from build123d import *

# Parameters (mm, degrees)
BOSS_EXTRUDE1_DEPTH = 20
SKETCH2_R           = 1.9
CUT_EXTRUDE1_DEPTH  = 7.5
CUT_EXTRUDE2_START  = -7.5
SKETCH3_R           = 1.9
CUT_EXTRUDE2_DEPTH  = 7.5


with BuildPart() as part:
    # Sketch1 → Boss-Extrude1 (new body)
    with BuildSketch(Plane(origin=(0, 0, 0), x_dir=(1, 0, 0), z_dir=(0, 1, 0))):
        Polygon((1.231025405, -2.055580158), (2.395697339, 0.038309195), (1.164671934, 2.093889353), (-1.231025405, 2.055580158), (-2.395697339, -0.038309195), (-1.164671934, -2.093889353), align=None)
    extrude(amount=BOSS_EXTRUDE1_DEPTH)

    # Sketch2 → Cut-Extrude1 (cut)
    with BuildSketch(Plane(origin=(0, 20, 0), x_dir=(1, 0, 0), z_dir=(0, 1, 0))):
        with Locations(Location((0, 0, 0), (0, 0, 270))):
            Circle(SKETCH2_R)
    extrude(amount=-CUT_EXTRUDE1_DEPTH, mode=Mode.SUBTRACT)

    # Sketch3 → Cut-Extrude2 (cut)
    with BuildSketch(Plane.XZ.offset(CUT_EXTRUDE2_START)):
        with Locations(Location((0, 0, 0), (0, 0, 90))):
            Circle(SKETCH3_R)
    extrude(amount=CUT_EXTRUDE2_DEPTH, mode=Mode.SUBTRACT)


solid = part.part
Source: CAD feature listing. Evaluate the final solid. Frame: model axes, mm. A direction names the side the tool comes from. Round coordinates to 2 decimals unless told otherwise and drop trailing zeros. Order: outer loops, then holes, each group sorted by start corner. A loop starts at its lowest first (then second) coordinate and runs counter-clockwise, first axis right, second up. Notation, with made-up numbers: (88.5, -32.75) - (109.5, -32.75) arc R23 cw to (109.5, -21.75) - close; hole circle Ø10 at (-20.5, 16.25). An arc over 180 degrees is marked (long way). Use a Markdown table: item, result. Add a question column.
1. Set-up query: faces 5 (the cylindrical face through (0.728, 3.802, 1.755)), 6 (the flat face through (-1.805, 9.86, -1.023)), 7 (the flat face through (0, 12.5, 0)). Return all of +Z, -Z, +X, -X, +Y, -Y with unobstructed straight access to the full face (end or side cutting, diameter ignored); none if empty.
2. Section query B-B (z = -1). Return the cut outline in (x, y).
3. Section query A-A (y = 17.75). Return the cut outline in (x, z).
4. Line query: probe 1 along Y at (x, z) = (-1, 0.1); probe 2 along X at (y, z) = (17, 0); probe 3 along X at (y, z) = (15.5, 0.35). Output: solid intervals per line, ascending.
5. Section query D-D (y = 10). Return the cut outline in (x, z).
6. Mould query, pull axis Z, two halves, no side actions, for faces 1 (the flat face through (0, 7.5, 0)), 2 (the flat face through (1.79, 9.86, -1.05)), 3 (the cylindrical face through (-0.728, 16.303, 1.755)), 4 (the flat face through (-1.79, 9.86, 1.05)). Classes: +Z half, -Z half, draft (parallel to the pull), parting line (faces both ways), or undercut.
7. Section query C-C (x = -0.75). Return the cut outline in (y, z).
8. First-contact query: pin 1 (1 mm diameter, centred on x = -0.5, y = 9.5, fed in from -Z); pin 2 (1.5 mm diameter, centred on y = 14.5, z = 1.5, fed in from -X). Flat tips, straight axial feed; report the tip coordinate or a pass-through.
Derived:
| question | item | result |
|---|---|---|
| 1 | face 5 | -Y |
| 1 | face 6 | -Z, -X, +Y, -Y |
| 1 | face 7 | +Y |
| 2 | outline | (-1.82, 0) - (-1.62, 0) - (-1.62, 7.5) - (1.62, 7.5) - (1.62, 0) - (1.82, 0) - (1.82, 20) - (1.62, 20) - (1.62, 12.5) - (-1.62, 12.5) - (-1.62, 20) - (-1.82, 20) - close |
| 3 | outline | (-2.4, 0.04) - (-1.23, -2.06) - (1.16, -2.09) - (2.4, -0.04) - (1.23, 2.06) - (-1.16, 2.09) - close; hole circle Ø3.8 at (0, 0) |
| 4 | probe 1 | 7.5 to 12.5 |
| 4 | probe 2 | -2.37 to -1.9, 1.9 to 2.37 |
| 4 | probe 3 | -2.21 to -1.87, 1.87 to 2.18 |
| 5 | outline | (-2.4, 0.04) - (-1.23, -2.06) - (1.16, -2.09) - (2.4, -0.04) - (1.23, 2.06) - (-1.16, 2.09) - close |
| 6 | face 1 | undercut |
| 6 | face 2 | -Z half |
| 6 | face 3 | undercut |
| 6 | face 4 | +Z half |
| 7 | outline | (0, -2.06) - (20, -2.06) - (20, -1.75) - (12.5, -1.75) - (12.5, 1.75) - (20, 1.75) - (20, 2.09) - (0, 2.09) - (0, 1.75) - (7.5, 1.75) - (7.5, -1.75) - (0, -1.75) - close |
| 8 | pin 1 | z = -2.08 |
| 8 | pin 2 | x = -1.97 |
